Design review of the part built by this model. Coordinates are the model's own, in mm. A direction names the side the tool comes from. Coordinates: 2 decimals unless noted, no trailing zeros. Loops run counter-clockwise (first coordinate to the right, second up) from the corner with the lowest first, then second, coordinate; pieces in that order, holes last. Notation, with made-up numbers: M -36,83 L 10,83 A9 ccw 10,95 Z; hole C 87,-35 d5. An arc over 180 degrees is marked long. Put each result on its own line as item: value. Start each with the question number.
(1) For faces 1 (the cylindrical face through (-863.81, -175.2, 4.44)), 2 (the flat face through (-899.722, -166.362, 4.437)), 3 (the flat face through (-819.92, -70.8, 4.44)), 4 (the cylindrical face through (-829.72, -57.91, 1.48)), list the 3-axis set-ups (+Z, -Z, +X, -X, +Y, -Y) from which the entire face can be reached by the end or side of a thin tool; tool diameter is ignored.
(2) Take a section at D-D, the plane x = -889. Give the boundary of the cut face in (y, z).
(3) Take a section at A-A, the plane x = -836. Give the boundary of the cut face in (y, z).
(4) For probe 1 along Y at (x, z) = (-826.5, 8.75); probe 2 along Y at (x, z) = (-827, 1.5); probe 3 along Z at (x, y) = (-828, -61.5), list the stretches that pass through material, from the lowest coordinate up. Write a range as [from, to].
(5) Take a section at C-C, the plane y = -142. Give the boundary of the cut face in (x, z).
(6) Take a section at B-B, the plane z = 4.5. Count the separate pieces of the cut face and the enclosed holes in it, then the cut area to 3 significant figures.
(7) Clearance check with flat-ended pins moving along their axes: pin 1 (5 mm diameter, centred on y = -112, z = 3, fed in from +X); pin 2 (1 mm diameter, centred on x = -855.5, z = 5.5, fed in from -Y); pin 3 (1 mm diameter, centred on x = -821.5, z = 5, fed in from -Y). State where each tip first meets the part, or that it passes through.
```python
from build123d import *

# Parameters (mm, degrees)
SKETCH2_R           = 2
SKETCH2_R_2         = 6.5
BOSS_EXTRUDE2_DEPTH = 9
BOSS_EXTRUDE5_START = 3
SKETCH2_7_R         = 6.5
SKETCH2_7_R_2       = 4
BOSS_EXTRUDE5_DEPTH = 3


with BuildPart() as part:
    # Sketch2 → Boss-Extrude2 (new body)
    with BuildSketch(Plane.XY):
        with BuildLine():
            Line((-793.550395835, -73.420672293), (-815.334160836, -55.043578334))
            ThreePointArc((-815.334160836, -55.043578334), (-829.724521088, -52.716019141), (-825.006315551, -66.508717808))
            Line((-825.006315551, -66.508717808), (-814.687690024, -75.213657052))
            Line((-814.687690024, -75.213657052), (-877.556695674, -149.737063634))
            ThreePointArc((-877.556695674, -149.737063634), (-884.354900869, -153.253176529), (-891.648225133, -150.932386807))
            Line((-891.648225133, -150.932386807), (-892.030396449, -150.609981649))
            ThreePointArc((-892.030396449, -150.609981649), (-893.489061302, -150.145823705), (-894.848702341, -150.849046284))
            Line((-894.848702341, -150.849046284), (-905.810477685, -163.842871021))
            ThreePointArc((-905.810477685, -163.842871021), (-907.202951518, -168.21886558), (-905.093283782, -172.297788697))
            Line((-905.093283782, -172.297788697), (-883.691690097, -190.352477499))
            ThreePointArc((-883.691690097, -190.352477499), (-879.315695538, -191.744951332), (-875.236772421, -189.635283596))
            Line((-875.236772421, -189.635283596), (-864.274997077, -176.641458858))
            ThreePointArc((-864.274997077, -176.641458858), (-863.810839132, -175.182794005), (-864.514061711, -173.823152966))
            Line((-864.514061711, -173.823152966), (-864.896233027, -173.500747809))
            ThreePointArc((-864.896233027, -173.500747809), (-868.412345922, -166.702542614), (-866.0915562, -159.409218349))
            Line((-866.0915562, -159.409218349), (-793.550395835, -73.420672293))
        make_face()
        Polygon((-898.215030346, -167.633870852), (-901.272400872, -165.054629594), (-899.337969929, -162.761601699), (-896.280599403, -165.340842957), align=None, mode=Mode.SUBTRACT)
        Polygon((-877.195607976, -185.366154496), (-880.252978503, -182.786913239), (-878.31854756, -180.493885344), (-875.261177033, -183.073126602), align=None, mode=Mode.SUBTRACT)
        with Locations((-868.600074365, -150.751427834)):
            Circle(SKETCH2_R, mode=Mode.SUBTRACT)
        with Locations((-836.359558647, -112.534296253)):
            Circle(SKETCH2_R, mode=Mode.SUBTRACT)
        with Locations((-823.46335236, -97.247443621)):
            Circle(SKETCH2_R, mode=Mode.SUBTRACT)
        with Locations((-804.119042929, -74.317164672)):
            Circle(SKETCH2_R, mode=Mode.SUBTRACT)
        with Locations((-823.22760872, -58.196906813)):
            Circle(SKETCH2_R_2, mode=Mode.SUBTRACT)
    extrude(amount=BOSS_EXTRUDE2_DEPTH)

    # Sketch2<7> → Boss-Extrude5 (add)
    with BuildSketch(Plane.XY.offset(BOSS_EXTRUDE5_START)):
        with Locations((-823.22760872, -58.196906813)):
            Circle(SKETCH2_7_R)
        with Locations((-823.22760872, -58.196906813)):
            Circle(SKETCH2_7_R_2, mode=Mode.SUBTRACT)
    extrude(amount=BOSS_EXTRUDE5_DEPTH)


solid = part.part
```
Computed values:
1. face 1: +Z, -Z, +X
1. face 2: +Z, -Z
1. face 3: +Z, -Z, -X
1. face 4: -Z
2. outline: M -185.87,0 L -152.54,0 L -152.54,9 L -185.87,9 Z
3. outline: M -123.74,0 L -114.5,0 L -114.5,9 L -123.74,9 Z; M -110.57,0 L -100.48,0 L -100.48,9 L -110.57,9 Z
4. probe 1: y = [-112.48, -89.22], [-66.04, -63.81], [-52.58, -50.35]
4. probe 2: y = [-113.07, -89.81], [-65.81, -63.49], [-52.9, -50.58]
4. probe 3: z = [3, 6]
5. outline: M -871.03,0 L -851.4,0 L -851.4,9 L -871.03,9 Z
6. separate pieces: 1
6. enclosed holes: 7
6. area: 3,120 mm^2
7. pin 1: stops at x = -823.99
7. pin 2: stops at y = -147.45
7. pin 3: stops at y = -107.14
